Verification items for this drawing (mm, ordinates from the low corner). Coordinates: 2 decimals unless noted, no trailing zeros. Write each loop counter-clockwise with the first axis right and the second up, starting at its lowest first coordinate (ties: lowest second). Pieces come first, ordered by that corner, then holes. Notation, with made-up numbers: (82.5, 46.25) -> (116.5, 46.25) arc R9 ccw to (116.5, 50.25) -> close; hole circle Ø2 at (14, -11). An arc over 180 degrees is marked (long way). One line per question, with ' | ' between items.
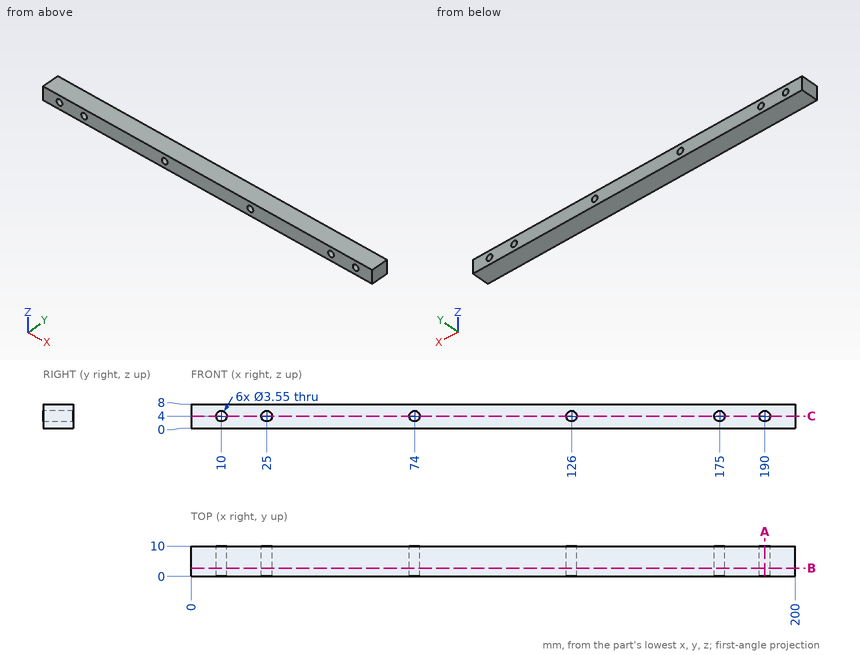
(1) Cross-section at B-B (y = 2.75). Record the cut outline in (x, z) (3 decimals).
Answers below:
outline: (0, 0) -> (200, 0) -> (200, 8) -> (0, 8) -> close; hole circle Ø3.55 at (10, 4); hole circle Ø3.55 at (25, 4); hole circle Ø3.55 at (74, 4); hole circle Ø3.55 at (126, 4); hole circle Ø3.55 at (175, 4); hole circle Ø3.55 at (190, 4)
(2) Depth check by flat-ended pin: P1, Ø3, axis at x = 126, z = 4, coming from the +Y side (3 decimals). Enter the tip coordinate at first touch or a pass-through.
Answers below:
P1: passes through
(3) Material ranges on line 1 (Z direction, x = 74, y = 2.25) (3 decimals), recorded low to high.
Answers below:
line 1: z = 0 to 2.225, 5.775 to 8
(4) Cross-section at A-A (x = 190). Record the cut outline in (y, z) (3 decimals).
Answers below:
outline: (0, 0) -> (10, 0) -> (10, 2.225) -> (0, 2.225) -> close; (0, 5.775) -> (10, 5.775) -> (10, 8) -> (0, 8) -> close
(5) Cross-section at C-C (z = 4). Record the cut outline in (x, y) (3 decimals).
Answers below:
outline: (0, 0) -> (8.225, 0) -> (8.225, 10) -> (0, 10) -> close; (11.775, 0) -> (23.225, 0) -> (23.225, 10) -> (11.775, 10) -> close; (26.775, 0) -> (72.225, 0) -> (72.225, 10) -> (26.775, 10) -> close; (75.775, 0) -> (124.225, 0) -> (124.225, 10) -> (75.775, 10) -> close; (127.775, 0) -> (173.225, 0) -> (173.225, 10) -> (127.775, 10) -> close; (176.775, 0) -> (188.225, 0) -> (188.225, 10) -> (176.775, 10) -> close; (191.775, 0) -> (200, 0) -> (200, 10) -> (191.775, 10) -> close
